```python
from build123d import *

# Parameters (mm, degrees)
SKETCH_R     = 1.5
PAD_DEPTH    = 1.6
SKETCH001_W  = 24.91
SKETCH001_H  = 15
PAD001_DEPTH = 1.75
SKETCH002_W  = 20
SKETCH002_H  = 8
PAD002_DEPTH = 5.5


with BuildPart() as part:
    # Sketch → Pad (new body)
    with BuildSketch(Plane.XY):
        with BuildLine():
            ThreePointArc((-15, 16), (-16.767767, 15.267767), (-17.5, 13.5))
            Line((-17.5, 13.5), (-17.5, -13.5))
            ThreePointArc((-17.5, -13.5), (-16.767767, -15.267767), (-15, -16))
            Line((-15, -16), (15, -16))
            ThreePointArc((15, -16), (16.767767, -15.267767), (17.5, -13.5))
            Line((17.5, 13.5), (17.5, -13.5))
            ThreePointArc((17.5, 13.5), (16.767767, 15.267767), (15, 16))
            Line((-15, 16), (15, 16))
        make_face()
        with Locations((-15, 13.5)):
            Circle(SKETCH_R, mode=Mode.SUBTRACT)
        with Locations((15, 13.5)):
            Circle(SKETCH_R, mode=Mode.SUBTRACT)
        with Locations((15, -13.5)):
            Circle(SKETCH_R, mode=Mode.SUBTRACT)
        with Locations((-15, -13.5)):
            Circle(SKETCH_R, mode=Mode.SUBTRACT)
    extrude(amount=PAD_DEPTH)

    # Sketch001 → Pad001 (join)
    with BuildSketch(Plane.XY.offset(1.6)):
        with Locations((-3.045, 0)):
            Rectangle(SKETCH001_W, SKETCH001_H)
    extrude(amount=PAD001_DEPTH)

    # Sketch002 → Pad002 (join)
    with BuildSketch(Plane.XY):
        with Locations((0, -12)):
            Rectangle(SKETCH002_W, SKETCH002_H)
    extrude(amount=-PAD002_DEPTH)


solid = part.part
```
For this review, take the finished solid that the model builds, in its own axes (mm). A direction names the side the tool comes from. Give positions to 0.01 mm unless a question says otherwise; leave off trailing zeros. Write each loop counter-clockwise with the first axis right and the second up, starting at its lowest first coordinate (ties: lowest second). Pieces come first, ordered by that corner, then holes.
Item 1: Take a section at B-B (x = -14). Give the boundary of the cut face in (y, z).
Item 2: Insertion check: P1, Ø12, axis at x = -9, y = 10.5, coming from the -Z side; P2, Ø1.5, axis at x = 4.5, y = 11, coming from the +Z side; P3, Ø1.6, axis at y = -12, z = -3.5, coming from the +X side. Each pin has a flat end and moves straight along its axis. Give the tip position at first contact, or say it passes through.
Item 3: Machinability: for faces 4 (the face through (-3, 7.5, 2)), 5 (the face through (10, -12, -3)), 6 (the face through (-15.5, 0, 2)), 7 (the face through (-3, -7.5, 2)), 8 (the face through (-10, -12, -3)), which of the approach directions +Z, -Z, +X, -X, +Y, -Y give a long, thin tool a straight path to every point of the face, cutting with its end or side? Answer none if there is none.
Item 4: Take a section at D-D (y = 7). Give the boundary of the cut face in (x, z).
Item 5: The part is to be moulded in two halves that separate along Y. For faces 1 (the face through (-17.5, 0, 1)), 2 (the face through (-17, 15, 1)), 3 (the face through (-16.5, -13.43, 0.79)), say which applies: +Y half, -Y half, draft (parallel to the pull), parting line (faces both ways), or undercut.
Item 6: Take a section at C-C (x = -4). Give the boundary of the cut face in (y, z), and give its area (3 significant figures).
Item 7: Wall thickness on probe 1 along Y at (x, z) = (15, 1); probe 2 along Z at (x, y) = (1, 14); probe 3 along Y at (x, z) = (4.5, 2.5): over which ranges is each line inside the solid? List them lowest first.
Item 8: Take a section at A-A (z = 0.75). Give the boundary of the cut face in (x, y).
Established:
1. outline: (-16, 0) - (-14.62, 0) - (-14.62, 1.6) - (-16, 1.6) - close; (-12.38, 0) - (12.38, 0) - (12.38, 1.6) - (7.5, 1.6) - (7.5, 3.35) - (-7.5, 3.35) - (-7.5, 1.6) - (-12.38, 1.6) - close; (14.62, 0) - (16, 0) - (16, 1.6) - (14.62, 1.6) - close
2. P1: stops at z = 0
2. P2: stops at z = 1.6
2. P3: stops at x = 10
3. face 4: +Z, +X, -X, +Y
3. face 5: -Z, +X, +Y, -Y
3. face 6: +Z, -X, +Y, -Y
3. face 7: +Z, +X, -X, -Y
3. face 8: -Z, -X, +Y, -Y
4. outline: (-17.5, 0) - (17.5, 0) - (17.5, 1.6) - (9.41, 1.6) - (9.41, 3.35) - (-15.5, 3.35) - (-15.5, 1.6) - (-17.5, 1.6) - close
5. face 1: draft
5. face 2: +Y half
5. face 3: undercut
6. outline: (-16, -5.5) - (-8, -5.5) - (-8, 0) - (16, 0) - (16, 1.6) - (7.5, 1.6) - (7.5, 3.35) - (-7.5, 3.35) - (-7.5, 1.6) - (-16, 1.6) - close
6. area: 121 mm2
7. probe 1: y = -16 to -15, -12 to 12, 15 to 16
7. probe 2: z = 0 to 1.6
7. probe 3: y = -7.5 to 7.5
8. outline: (-17.5, -13.5) arc R2.5 ccw to (-15, -16) - (15, -16) arc R2.5 ccw to (17.5, -13.5) - (17.5, 13.5) arc R2.5 ccw to (15, 16) - (-15, 16) arc R2.5 ccw to (-17.5, 13.5) - close; hole circle Ø3 at (-15, -13.5); hole circle Ø3 at (-15, 13.5); hole circle Ø3 at (15, -13.5); hole circle Ø3 at (15, 13.5)
